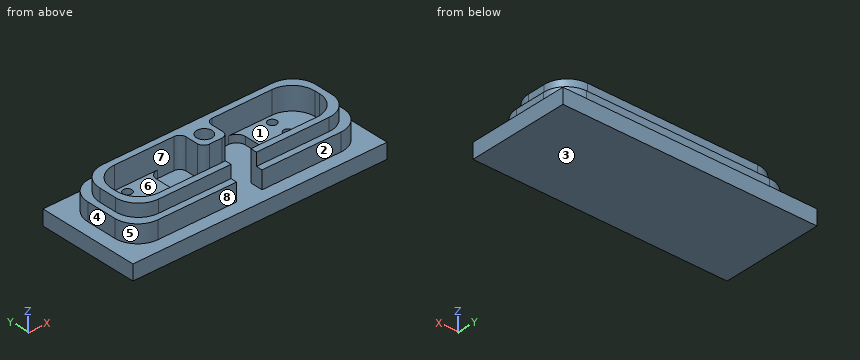
Autodesk Fusion 360 part; units mm, degrees
sketch "Sketch1" plane through (0, 0, 0) normal (0, 0, 1) x (1, 0, 0)
  line L0 (99.503, -40) -> (-100.497, -40)
  line L1 (-100.497, -40) -> (-100.497, 40)
  line L2 (-100.497, 40) -> (99.503, 40)
  line L3 (99.503, 40) -> (99.503, -40)
  line L4 (99.503, -40) -> (-100.497, 40) construction
  line L5 (-100.497, -40) -> (99.503, 40) construction
  point P0 (-0.497, 0)
  dimension "d1" = 200
  dimension "d2" = 80
extrude "Extrude1" add sketch "Sketch1" along normal blind 12
sketch "Sketch2" plane through (0, 0, 12) normal (0, 0, 1) x (-1, 0, 0)
  line L0 (-99.503, -40) -> (100.497, -40)
  line L1 (100.497, -40) -> (100.497, 40)
  line L2 (100.497, 40) -> (-99.503, 40)
  line L3 (-99.503, 40) -> (-99.503, -40)
  line L4 (90, -30) -> (-90, -30)
  line L5 (-90, -30) -> (-90, 30)
  line L6 (-90, 30) -> (-10, 30)
  line L7 (-10, 30) -> (-10, 20)
  line L8 (-10, 20) -> (-80, 20)
  line L9 (-80, 20) -> (-80, -20)
  line L10 (-80, -20) -> (80, -20)
  line L11 (80, -20) -> (80, 20)
  line L12 (80, 20) -> (10, 20)
  line L13 (10, 30) -> (10, 20)
  line L14 (10, 30) -> (90, 30)
  line L15 (90, 30) -> (90, -30)
  line L16 (10, 25) -> (85, 25)
  line L17 (85, 25) -> (85, -25)
  line L18 (85, -25) -> (10, -25)
  line L19 (10, -25) -> (10, 0)
  line L20 (10, 0) -> (-10, 0)
  line L21 (-10, 0) -> (-10, -25)
  line L22 (-10, -25) -> (-85, -25)
  line L23 (-85, -25) -> (-85, 25)
  line L24 (-85, 25) -> (-10, 25)
  line L25 (10, -25) -> (-10, -25)
extrude "Extrude2" add sketch "Sketch2" along normal blind 15 contours L10 L11 L12 L13 L16 L17 L18 L19 | L7 L8 L9 L10 L21 L22 L23 L24 | L10 L19 L21 L25 | L10 L19 L20 L21
sketch "Sketch3" plane through (0, 0, 12) normal (0, 0, 1) x (-1, 0, 0)
  line L0 (10, 25) -> (85, 25)
  line L1 (85, 25) -> (85, -25)
  line L2 (85, -25) -> (-85, -25)
  line L3 (-85, -25) -> (-85, 25)
  line L4 (-85, 25) -> (-10, 25)
  line L5 (-10, 25) -> (-10, 20)
  line L6 (-10, 20) -> (-80, 20)
  line L7 (-80, 20) -> (-80, -20)
  line L8 (-80, -20) -> (-10, -20)
  line L9 (-10, -20) -> (-10, 0)
  line L10 (-10, 0) -> (10, 0)
  line L11 (10, 0) -> (10, -20)
  line L12 (10, -20) -> (80, -20)
  line L13 (80, -20) -> (80, 20)
  line L14 (80, 20) -> (10, 20)
  line L15 (10, 20) -> (10, 25)
  line L16 (-99.503, -40) -> (100.497, -40)
  line L17 (100.497, -40) -> (100.497, 40)
  line L18 (100.497, 40) -> (-99.503, 40)
  line L19 (-99.503, 40) -> (-99.503, -40)
  line L20 (90, -30) -> (-90, -30)
  line L21 (-90, -30) -> (-90, 30)
  line L22 (-90, 30) -> (-10, 30)
  line L23 (-10, 30) -> (-10, 25)
  line L24 (10, 25) -> (10, 30)
  line L25 (10, 30) -> (90, 30)
  line L26 (90, 30) -> (90, -30)
extrude "Extrude3" add sketch "Sketch3" along normal blind 14 contours L0 L1 L2 L3 L4 L20 L21 L22 L23 L24 L25 L26
extrude "Extrude4" add 1 faces at (3.3333, 6.6667, 27) along direction (0, 0, 1) blind 9
fillet "Fillet1" radius 5 2 edges at (-10, 0, 24) (10, 0, 24)
fillet "Fillet2" radius 5 2 edges at (10, 20, 24) (-10, 20, 24)
fillet "Fillet3" radius 18 12 edges at (-85, -25, 31) (-90, -30, 19) (85, -25, 31) (90, -30, 19) (90, 30, 19) (85, 25, 31) (-90, 30, 19) (-85, 25, 31) (-80, 20, 24) (80, 20, 24) (-80, -20, 24) (80, -20, 24)
sketch "Sketch4" plane through (0, 0, 36) normal (0, 0, 1) x (-1, 0, 0)
  arc A0 (67, -25) -> (85, -7) centre (67, -7) ccw
  line L0 (85, -7) -> (85, 7)
  arc A1 (85, 7) -> (67, 25) centre (67, 7) ccw
  line L1 (67, 25) -> (10, 25)
  line L2 (10, 25) -> (10, 20)
  line L3 (10, 20) -> (62, 20)
  arc A2 (80, 2) -> (62, 20) centre (62, 2) ccw
  line L4 (80, 2) -> (80, -2)
  arc A3 (62, -20) -> (80, -2) centre (62, -2) ccw
  line L5 (62, -20) -> (15, -20)
  arc A4 (10, -15) -> (15, -20) centre (15, -15) ccw
  line L6 (10, -15) -> (10, -5)
  arc A5 (10, -5) -> (5, 0) centre (5, -5) ccw
  line L7 (5, 0) -> (-5, 0)
  arc A6 (-5, 0) -> (-10, -5) centre (-5, -5) ccw
  line L8 (-10, -5) -> (-10, -15)
  arc A7 (-15, -20) -> (-10, -15) centre (-15, -15) ccw
  line L9 (-15, -20) -> (-62, -20)
  arc A8 (-80, -2) -> (-62, -20) centre (-62, -2) ccw
  line L10 (-80, -2) -> (-80, 2)
  arc A9 (-62, 20) -> (-80, 2) centre (-62, 2) ccw
  line L11 (-62, 20) -> (-10, 20)
  line L12 (-10, 20) -> (-10, 25)
  line L13 (-10, 25) -> (-67, 25)
  arc A10 (-67, 25) -> (-85, 7) centre (-67, 7) ccw
  line L14 (-85, 7) -> (-85, -7)
  arc A11 (-85, -7) -> (-67, -25) centre (-67, -7) ccw
  line L15 (-67, -25) -> (67, -25)
  circle A12 centre (0, -10) radius 6.1104
extrude "Extrude5" cut sketch "Sketch4" against normal blind 30 contours A12
sketch "Sketch5" plane through (0, 0, 12) normal (0, 0, 1) x (-1, 0, 0)
  arc A0 (-62, 20) -> (-80, 2) centre (-62, 2) ccw
  line L0 (-80, 2) -> (-80, -2)
  arc A1 (-80, -2) -> (-62, -20) centre (-62, -2) ccw
  line L1 (-62, -20) -> (-15, -20)
  arc A2 (-15, -20) -> (-10, -15) centre (-15, -15) ccw
  line L2 (-10, -15) -> (-10, -5)
  arc A3 (-5, 0) -> (-10, -5) centre (-5, -5) ccw
  line L3 (-5, 0) -> (5, 0)
  arc A4 (10, -5) -> (5, 0) centre (5, -5) ccw
  line L4 (10, -5) -> (10, -15)
  arc A5 (10, -15) -> (15, -20) centre (15, -15) ccw
  line L5 (15, -20) -> (62, -20)
  arc A6 (62, -20) -> (80, -2) centre (62, -2) ccw
  line L6 (80, -2) -> (80, 2)
  arc A7 (80, 2) -> (62, 20) centre (62, 2) ccw
  line L7 (62, 20) -> (10, 20)
  line L8 (10, 20) -> (10, 30)
  line L9 (10, 30) -> (72, 30)
  arc A8 (90, 12) -> (72, 30) centre (72, 12) ccw
  line L10 (90, 12) -> (90, -12)
  arc A9 (72, -30) -> (90, -12) centre (72, -12) ccw
  line L11 (72, -30) -> (-72, -30)
  arc A10 (-90, -12) -> (-72, -30) centre (-72, -12) ccw
  line L12 (-90, -12) -> (-90, 12)
  arc A11 (-72, 30) -> (-90, 12) centre (-72, 12) ccw
  line L13 (-72, 30) -> (-10, 30)
  line L14 (-10, 30) -> (-10, 20)
  line L15 (-10, 20) -> (-62, 20)
  line L16 (-99.503, -40) -> (100.497, -40)
  line L17 (100.497, -40) -> (100.497, 40)
  line L18 (100.497, 40) -> (-99.503, 40)
  line L19 (-99.503, 40) -> (-99.503, -40)
  line L20 (35, 20) -> (35, -20)
  line L21 (-35, 20) -> (-35, -20)
extrude "Extrude6" add sketch "Sketch5" along normal blind 6 contours A0 L0 A1 L1 L15 L21 | L5 A6 L6 A7 L7 L20
fillet "Fillet4" radius 7 4 edges at (-35, 20, 15) (35, 20, 15) (35, -20, 15) (-35, -20, 15)
sketch "Sketch6" plane through (0, 0, 18) normal (0, 0, 1) x (-1, 0, 0)
  line L0 (35, 13) -> (35, -13)
  arc A0 (28, -20) -> (35, -13) centre (28, -13) ccw
  line L1 (28, -20) -> (62, -20)
  arc A1 (62, -20) -> (80, -2) centre (62, -2) ccw
  line L2 (80, -2) -> (80, 2)
  arc A2 (80, 2) -> (62, 20) centre (62, 2) ccw
  line L3 (62, 20) -> (28, 20)
  arc A3 (35, 13) -> (28, 20) centre (28, 13) ccw
  circle A4 centre (57, 0) radius 3.5
  circle A5 centre (57, 13) radius 3.5
  circle A6 centre (57, -14) radius 3.5
  dimension "d23" = 7
  dimension "d24" = 7
  dimension "d25" = 7
sketch "Sketch7" plane through (0, 0, 18) normal (0, 0, 1) x (-1, 0, 0)
  arc A0 (-62, 20) -> (-80, 2) centre (-62, 2) ccw
  line L0 (-80, 2) -> (-80, -2)
  arc A1 (-80, -2) -> (-62, -20) centre (-62, -2) ccw
  line L1 (-62, -20) -> (-28, -20)
  arc A2 (-35, -13) -> (-28, -20) centre (-28, -13) ccw
  line L2 (-35, -13) -> (-35, 13)
  arc A3 (-28, 20) -> (-35, 13) centre (-28, 13) ccw
  line L3 (-28, 20) -> (-62, 20)
  circle A4 centre (-57, 0) radius 3.5
  circle A5 centre (-57, -14) radius 3.5
  circle A6 centre (-57, 13) radius 3.5
  dimension "d26" = 7
  dimension "d27" = 7
  dimension "d28" = 7
extrude "Extrude7" cut sketch "Sketch7" sketch "Sketch6" against normal blind 10 contours A4 | A5 | A6 of sketch 2 contours A4 | A5 | A6
The listing builds one solid part. Answer for the finished solid, in the listing's coordinates (mm). Face numbers are marked on the shaded views. A direction names the side the tool comes from. Round coordinates to 2 decimals unless told otherwise and drop trailing zeros. Loops run counter-clockwise (first coordinate to the right, second up) from the corner with the lowest first, then second, coordinate; pieces in that order, holes last.
Q1. For a pull along X with two mould halves and no side action, classify the marked faces 5, 6, 7 and 8 as released by +X, released by -X, zero draft, split by the parting line, or undercut.
Q2. Section B-B, the plane y = 27.5 is taken. Determine the outline of the cut face in (x, z), then the cut area to 3 significant figures.
Q3. Section A-A, the plane x = -18.5 is taken. Determine the outline of the cut face in (y, z), then the cut area to 3 significant figures.
Q4. Given pin 1 Ø6 at (y, z) = (-5.5, 16) entering from +X; pin 2 Ø1 at (y, z) = (-20, 14.5) entering from +X; pin 3 Ø7 at (x, z) = (25.5, 28) entering from +Y, each flat-ended and moving along its own axis, determine where each tip first touches the part or whether it passes through.
Q5. Which of the six approach directions +Z, -Z, +X, -X, +Y, -Y give full straight-line access (tool end or side, diameter ignored) to the marked faces 1, 2, 3 and 4?
Q6. Find the intervals of material crossed by line 1 (Y direction, x = 57, z = 15); line 2 (X direction, y = 16.5, z = 17); line 3 (X direction, y = -13, z = 13), in increasing order.
Q7. Section C-C, the plane x = 75 is taken. Determine the outline of the cut face in (y, z), then the cut area to 3 significant figures.
Completed:
1. face 5: released by -X
1. face 6: undercut
1. face 7: undercut
1. face 8: zero draft
2. outline: (-100.5, 0) - (99.5, 0) - (99.5, 12) - (81.15, 12) - (81.15, 26) - (-81.15, 26) - (-81.15, 12) - (-100.5, 12) - close
2. area: 4,670 mm2
3. outline: (-40, 0) - (40, 0) - (40, 12) - (30, 12) - (30, 26) - (25, 26) - (25, 36) - (20, 36) - (20, 12) - (-20, 12) - (-20, 36) - (-25, 36) - (-25, 26) - (-30, 26) - (-30, 12) - (-40, 12) - close
3. area: 1,340 mm2
4. pin 1: stops at x = 90
4. pin 2: stops at x = 88.36
4. pin 3: stops at y = 30
5. face 1: +Z
5. face 2: +Z, +X, -X, -Y
5. face 3: -Z, +X, -X, +Y, -Y
5. face 4: +Z, -X, +Y, -Y
6. line 1: y = -30 to -16.5, -9.5 to -3.5, 3.5 to 10.5, 17.5 to 30
6. line 2: x = -89.43 to -59.45, -54.55 to -34.06, -10.23 to 10.23, 34.06 to 54.55, 59.45 to 89.43
6. line 3: x = -89.97 to -60.5, -53.5 to -35, 35 to 53.5, 60.5 to 89.97
7. outline: (-40, 0) - (40, 0) - (40, 12) - (29.75, 12) - (29.75, 26) - (23.12, 26) - (23.12, 36) - (14.45, 36) - (14.45, 18) - (-14.45, 18) - (-14.45, 36) - (-23.12, 36) - (-23.12, 26) - (-29.75, 26) - (-29.75, 12) - (-40, 12) - close
7. area: 1,740 mm2
